Check sheet for the modelled part. Datum: model origin and axes. Units: mm. Round coordinates to 2 decimals unless told otherwise and drop trailing zeros. Write each loop counter-clockwise with the first axis right and the second up, starting at its lowest first coordinate (ties: lowest second). Pieces come first, ordered by that corner, then holes. Notation, with made-up numbers: (14, 56.25) - (42, 56.25) arc R34 ccw to (42, 92.25) - close; hole circle Ø5 at (31, 40.5). An arc over 180 degrees is marked (long way). Answer as a JSON object with one key per item and string values. Group by question number.
Item 1: Sectioned sample at A-A on y = 0. Record the boundary of the cut face in (x, z).
Item 2: Sectioned sample at B-B on z = 0. Record the boundary of the cut face in (x, y).
Item 3: Sectioned sample at C-C on x = 0. Record the boundary of the cut face in (y, z), plus the area to 3 significant figures.
Item 4: Sectioned sample at D-D on z = 3. Record the boundary of the cut face in (x, y).
Item 5: Gauge pin test, flat ends, axial feed: P1, Ø6, axis at x = -7, z = 1.5, coming from the +Y side; P2, Ø10, axis at x = -6, z = -11, coming from the +Y side; P3, Ø5, axis at x = 5, y = -9, coming from the +Z side; P4, Ø8, axis at y = 2, z = 4, coming from the +X side. Record the tip position at first contact, or that the pin passes through.
Item 6: Thickness scan on line 1 (Z direction, x = 1, y = 0.25); line 2 (Z direction, x = -3.75, y = -4.5); line 3 (Y direction, x = 4.5, z = 0). Record the ranges inside material, lowest first.
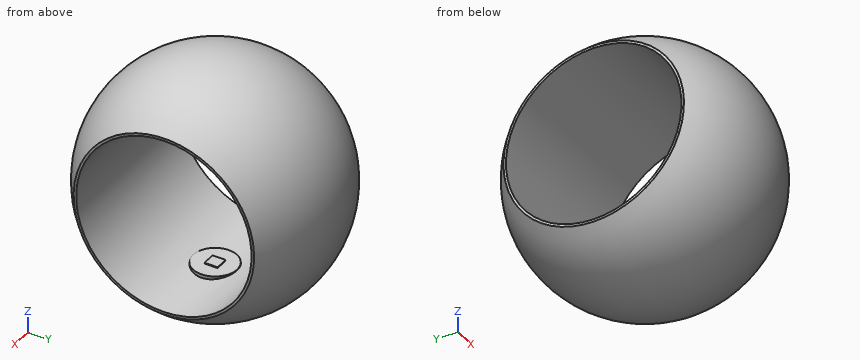
Autodesk Inventor part; units mm, degrees
ref_plane "Work Plane1" through (0, 0, -10) normal (0, 0, 1) x (1, 0, 0)
ref_plane "YZ Plane" through (0, 0, 0) normal (1, 0, 0) x (0, 1, 0)
ref_plane "XZ Plane" through (0, 0, 0) normal (0, 1, 0) x (-1, 0, 0)
sketch "Sketch1" plane through (0, 0, 0) normal (0, 1, 0) x (-1, 0, 0)
  line L0 (9.5, 0) -> (-9.5, 0)
  line L1 (9.5, 0) -> (9.5, -10) construction
  line L2 (-9.5, 0) -> (-9.5, -10) construction
  line L3 (9.5, -10) -> (9.5, -10.2835)
  line L4 (-9.5, -10) -> (-9.5, -10.2835)
  arc A0 (-9.5, -10.2835) -> (9.5, -10.2835) centre (0, 0) ccw
  line L5 (9.5, -10) -> (-9.5, -10)
  dimension "d0" = 19
  dimension "d7" = 14
  dimension "d9" = 10
ref_plane "Work Plane1" through (0, 0, -10) normal (0, 0, 1) x (1, 0, 0)
revolve "Revolution2" add sketch "Sketch1" angle 360 about axis through (-9.5, 0, 0) along (1, 0, 0)
sketch "Sketch4" plane through (0, 0, -10) normal (0, 0, 1) x (1, 0, 0)
  circle A0 centre (0, 0) radius 2.5
  dimension "d17" = 5
extrude "Extrusion3" add sketch "Sketch4" along normal blind 0.4
sketch "Sketch5" plane through (0, 0, -9.6) normal (0, 0, 1) x (1, 0, 0)
  circle A0 centre (0, 0) radius 2.5
  line L0 (0.75, 0.75) -> (0.75, -0.75)
  line L1 (0.75, -0.75) -> (-0.75, -0.75)
  line L2 (-0.75, -0.75) -> (-0.75, 0.75)
  line L3 (-0.75, 0.75) -> (0.75, 0.75)
  point P0 (0.5831, -2.431)
  point P1 (0.5831, 2.431)
  dimension "d20" = 1.5
extrude "Extrusion4" add sketch "Sketch5" along normal blind 0.1 contours L0 L1 L2 L3
properties part number "Smart Ring" material "Titanium"
Completed:
{
 "1": {"outline": "(-9.5, -10.28) arc R14 ccw to (9.5, -10.28) - (9.5, -10) - (2.5, -10) - (2.5, -9.6) - (0.75, -9.6) - (0.75, -9.5) - (-0.75, -9.5) - (-0.75, -9.6) - (-2.5, -9.6) - (-2.5, -10) - (-9.5, -10) - close; (-9.5, 10) - (9.5, 10) - (9.5, 10.28) arc R14 ccw to (-9.5, 10.28) - close"},
 "2": {"outline": "(-9.5, -10.28) arc R14 ccw to (9.5, -10.28) - (9.5, -10) - (-9.5, -10) - close; (-9.5, 10) - (9.5, 10) - (9.5, 10.28) arc R14 ccw to (-9.5, 10.28) - close"},
 "3": {"outline": "circle Ø28 at (0, 0); hole (-2.5, -9.68) - (-2.5, -9.6) - (-0.75, -9.6) - (-0.75, -9.5) - (0.75, -9.5) - (0.75, -9.6) - (2.5, -9.6) - (2.5, -9.68) arc R10 ccw (long way) to start", "area": "303 mm²"},
 "4": {"outline": "(-9.5, -9.84) arc R13.67 ccw to (9.5, -9.84) - (9.5, -9.54) - (-9.5, -9.54) - close; (-9.5, 9.54) - (9.5, 9.54) - (9.5, 9.84) arc R13.67 ccw to (-9.5, 9.84) - close"},
 "5": {"P1": "y = 13.37", "P2": "y = 11.8", "P3": "z = 11.63", "P4": "through"},
 "6": {"line 1": "-13.96 to -9.6, 10 to 13.96", "line 2": "-12.72 to -8.93, 8.93 to 12.72", "line 3": "-13.26 to -10, 10 to 13.26"}
}
